Autodesk Inventor part; units mm, degrees
ref_plane "YZ Plane" through (0, 0, 0) normal (1, 0, 0) x (0, 1, 0)
ref_plane "XZ Plane" through (0, 0, 0) normal (0, 1, 0) x (-1, 0, 0)
ref_plane "XY Plane" through (0, 0, 0) normal (0, 0, 1) x (1, 0, 0)
sketch "Sketch14" plane through (0, 0, 0) normal (0, 0, 1) x (1, 0, 0)
  line L0 (0, 0) -> (-20, 0)
  line L1 (-20, 0) -> (-20, 20)
  line L2 (-20, 20) -> (0, 20)
  line L3 (0, 20) -> (0, 0)
  line L4 (-5, 5) -> (-10, 5)
  line L5 (-10, 5) -> (-10, 10)
  line L6 (-10, 10) -> (-5, 10)
  line L7 (-5, 10) -> (-5, 5)
  dimension "d71" = 20
  dimension "d72" = 20
  dimension "d73" = 5
  dimension "d74" = 5
extrude "Extrusion9" add sketch "Sketch14" along normal blind 25 contours L0 L1 L2 L3 | L4 L5 L6 L7
fillet "Fillet1" radius 2 12 edges at (-20, 20, 12.5) (-20, 10, 0) (-20, 0, 12.5) (-20, 10, 25) (0, 10, 25) (-10, 20, 25) (0, 20, 12.5) (-10, 20, 0) (-10, 0, 25) (0, 10, 0) (0, 0, 12.5) (-10, 0, 0)
sketch "Sketch24" plane through (0, 0, 25) normal (0, 0, 1) x (1, 0, 0)
  line L0 (-15, 15) -> (-5, 15)
  line L1 (-5, 15) -> (-5, 5)
  line L2 (-5, 5) -> (-15, 5)
  line L3 (-15, 5) -> (-15, 15)
  point P0 (0, 0)
  dimension "d176" = 10
  dimension "d177" = 10
extrude "Extrusion16" cut sketch "Sketch24" against normal blind 10
sketch "Sketch31" plane through (0, 0, 0) normal (0, 0, -1) x (-1, 0, 0)
  line L0 (5, 5) -> (15, 5)
  line L1 (15, 5) -> (15, 15)
  line L2 (15, 15) -> (5, 15)
  line L3 (5, 15) -> (5, 5)
  point P0 (0, 0)
  dimension "d231" = 10
  dimension "d232" = 10
extrude "Extrusion18" cut sketch "Sketch31" against normal blind 10
chamfer "Chamfer15" distance 1 angle 45 8 edges at (-10, 15, 0) (-15, 10, 0) (-10, 5, 0) (-5, 10, 0) (-10, 15, 25) (-5, 10, 25) (-10, 5, 25) (-15, 10, 25)
properties part number "Hole_TestFits"
CAD build for the part. Positions are in the model's coordinates, mm. A direction names the side the tool comes from. Coordinates: 2 decimals unless noted, no trailing zeros. Loops run counter-clockwise (first coordinate to the right, second up) from the corner with the lowest first, then second, coordinate; pieces in that order, holes last. Notation, with made-up numbers: (-23, -37.5) -> (33, -37.5) arc R13 cw to (33, -18.5) -> close; hole circle Ø11 at (64, -25.5). An arc over 180 degrees is marked (long way). One line per item, written item: value.
1. Slice it at D-D on y = 1.5. Write the cut outline in (x, z), and give its area (3 significant figures).
Answers:
outline: (-19.94, 2) arc R1.94 ccw to (-18, 0.06) -> (-2, 0.06) arc R1.94 ccw to (-0.06, 2) -> (-0.06, 23) arc R1.94 ccw to (-2, 24.94) -> (-18, 24.94) arc R1.94 ccw to (-19.94, 23) -> close
area: 491 mm^2
2. Slice it at A-A on z = 16.5. Write the cut outline in (x, y), and give its area (3 significant figures).
Answers:
outline: (-20, 2) arc R2 ccw to (-18, 0) -> (-2, 0) arc R2 ccw to (0, 2) -> (0, 18) arc R2 ccw to (-2, 20) -> (-18, 20) arc R2 ccw to (-20, 18) -> close; hole (-15, 5) -> (-5, 5) -> (-5, 15) -> (-15, 15) -> close
area: 297 mm^2
3. Slice it at B-B on x = -12. Write the cut outline in (y, z), and give its area (3 significant figures).
Answers:
outline: (0, 2) arc R2 ccw to (2, 0) -> (4, 0) -> (5, 1) -> (5, 10) -> (15, 10) -> (15, 1) -> (16, 0) -> (18, 0) arc R2 ccw to (20, 2) -> (20, 23) arc R2 ccw to (18, 25) -> (16, 25) -> (15, 24) -> (15, 15) -> (5, 15) -> (5, 24) -> (4, 25) -> (2, 25) arc R2 ccw to (0, 23) -> close
area: 295 mm^2
4. Slice it at C-C on y = 11. Write the cut outline in (x, z), and give its area (3 significant figures).
Answers:
outline: (-20, 2) arc R2 ccw to (-18, 0) -> (-16, 0) -> (-15, 1) -> (-15, 10) -> (-5, 10) -> (-5, 1) -> (-4, 0) -> (-2, 0) arc R2 ccw to (0, 2) -> (0, 23) arc R2 ccw to (-2, 25) -> (-4, 25) -> (-5, 24) -> (-5, 15) -> (-15, 15) -> (-15, 24) -> (-16, 25) -> (-18, 25) arc R2 ccw to (-20, 23) -> close
area: 295 mm^2
5. Which spindle directions (+Z, -Z, +X, -X, +Y, -Y) get a long thin tool onto all of the face, cutting with end or side? Do faces 5 (the face through (-10, 15, 20)), 6 (the face through (-10, 10, 10)), 7 (the face through (-0.6, 0.57, 12.65)). Say none if no direction does.
Answers:
face 5: +Z
face 6: -Z
face 7: +Z, -Z, +X, -Y
6. Drill centre lines: line 1 (Y direction, x = -13.5, z = 20); line 2 (X direction, y = 12, z = 4.75); line 3 (Z direction, x = -6.75, y = 7). Where is each one in solid material? Low to high. Write a range as [from, to].
Answers:
line 1: y = [0, 5], [15, 20]
line 2: x = [-20, -15], [-5, 0]
line 3: z = [10, 15]
7. Pull direction Y, two halves, no side cores. Call faces 1 (the face through (-10, 5, 20)), 2 (the face through (-0.57, 19.4, 12.65)), 3 (the face through (-19.43, 0.6, 12.65)), 4 (the face through (-0.57, 9.89, 24.4)): pulls with the +Y half, pulls with the -Y half, needs draft (parallel to the pull), parting line crosses it, or undercut.
Answers:
face 1: undercut
face 2: pulls with the +Y half
face 3: pulls with the -Y half
face 4: needs draft
8. Flat gauge pins, fed straight in: P1, Ø10, axis at x = -13, y = 11.5, coming from the +Z side; P2, Ø1.5, axis at x = -10.5, y = 5, coming from the +Z side; P3, Ø3, axis at x = -12, y = 8, coming from the +Z side; P4, Ø5, axis at x = -8, y = 10, coming from the -Z side. Where does each tip first touch, or does it go through?
Answers:
P1: stops at z = 25
P2: stops at z = 24.75
P3: stops at z = 15
P4: stops at z = 10
